Check sheet for the modelled part. Datum: model origin and axes. Units: mm. Face numbers are marked on the shaded views. A direction names the side the tool comes from. Give positions to 0.01 mm unless a question says otherwise; leave off trailing zeros. Loops run counter-clockwise (first coordinate to the right, second up) from the corner with the lowest first, then second, coordinate; pieces in that order, holes last. Notation, with made-up numbers: (58.25, 53.25) -> (75.25, 53.25) arc R21 cw to (75.25, 75.25) -> close; hole circle Ø8 at (81.25, 9). An arc over 180 degrees is marked (long way). Write each question's results on one line, items separated by ' | '. Start each with the question number.
Item 1: Cross-section at D-D on x = 25. Enter the section's corners in (y, z), then the cut area to 3 significant figures.
Item 2: Cross-section at B-B on y = 9.5. Enter the section's corners in (x, z).
Item 3: Mould release check, pull along X, two halves, no side actions. Record for the marked faces 3, 4 and 5: pulls with the +X half, pulls with the -X half, needs draft (parallel to the pull), parting line crosses it, or undercut.
Item 4: Cross-section at C-C on x = -14.5. Enter the section's corners in (y, z), then the cut area to 3 significant figures.
Item 5: Gauge pin test, flat ends, axial feed: pin 1 Ø3 at (x, y) = (-13.5, -5) entering from -Z; pin 2 Ø12 at (x, y) = (-1.5, -8) entering from -Z. Record the tip position at first contact, or that the pin passes through.
Item 6: Access from +Z, -Z, +X, -X, +Y, -Y to the whole of each face (thin tool, end or side, straight path). Record for the marked faces 1 and 2.
Item 7: Cross-section at A-A on z = 18.25. Enter the section's corners in (x, y).
Item 8: Scan lines: line 1 along Y through (x, z) = (7.5, 23.5); line 2 along X through (y, z) = (-13, 14.75); line 3 along X through (y, z) = (-8.5, 16). Record each from-to range of solid material in increasing order.
from build123d import *

# Parameters (mm, degrees)
F0_W     = 70
F0_H     = 40
F1_DEPTH = 25
F3_DEPTH = 70.001


with BuildPart() as f1:
    # F0 (on Top) → F1 (new body)
    with BuildSketch(Plane.XY):
        Rectangle(F0_W, F0_H)
        Polygon((-8, -13.856406), (-16, 0), (-8, 13.856406), (8, 13.856406), (16, 0), (8, -13.856406), align=None, mode=Mode.SUBTRACT)
    extrude(amount=F1_DEPTH)

    # F2 (on face) → F3 (cut, through all)
    with BuildSketch(Plane.YZ.offset(35)):
        with BuildLine():
            ThreePointArc((-16.922921, 0), (0, -16.922921), (16.922921, 0))
            Line((16.922921, 0), (-16.922921, 0))
        make_face()
        with BuildLine():
            Line((-16.922921, 0), (16.922921, 0))
            ThreePointArc((16.922921, 0), (0, 16.922921), (-16.922921, 0))
        make_face()
    extrude(amount=-F3_DEPTH, mode=Mode.SUBTRACT)


solid = f1.part
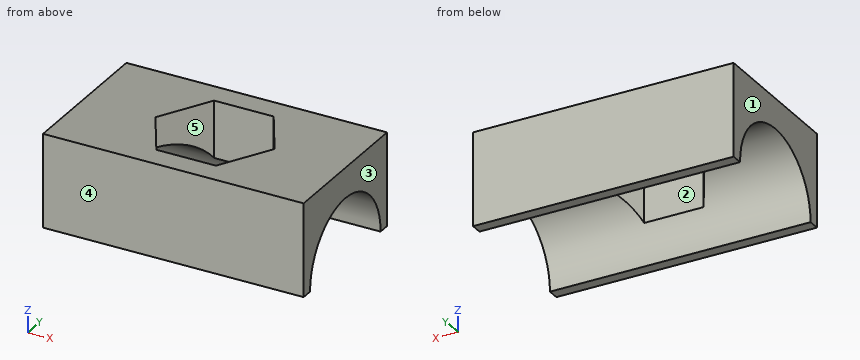
Answer sheet:
1) outline: (-20, 0) -> (-16.92, 0) arc R16.92 cw to (16.92, 0) -> (20, 0) -> (20, 25) -> (-20, 25) -> close | area: 550 mm²
2) outline: (-35, 14) -> (-10.52, 14) -> (-10.52, 25) -> (-35, 25) -> close; (10.52, 14) -> (35, 14) -> (35, 25) -> (10.52, 25) -> close
3) face 3: pulls with the +X half | face 4: needs draft | face 5: undercut
4) outline: (-20, 0) -> (-16.92, 0) arc R16.92 cw to (-2.6, 16.72) -> (-2.6, 25) -> (-20, 25) -> close; (2.6, 16.72) arc R16.92 cw to (16.92, 0) -> (20, 0) -> (20, 25) -> (2.6, 25) -> close | area: 508 mm²
5) pin 1: stops at z = 15.62 | pin 2: stops at z = 9.51
6) face 1: +Z, -Z, -X, +Y, -Y | face 2: +Z, -Z
7) outline: (-35, -20) -> (35, -20) -> (35, 20) -> (-35, 20) -> close; hole (-16, 0) -> (-8, -13.86) -> (8, -13.86) -> (16, 0) -> (8, 13.86) -> (-8, 13.86) -> close
8) line 1: y = -20 to -13.86, 13.86 to 20 | line 2: x = -35 to -8.49, 8.49 to 35 | line 3: x = -35 to -11.09, 11.09 to 35
